The model under review builds one solid part; all positions refer to its coordinate system, in mm. Give positions to 0.01 mm unless a question says otherwise; leave off trailing zeros. Loops run counter-clockwise (first coordinate to the right, second up) from the corner with the lowest first, then second, coordinate; pieces in that order, holes last. Notation, with made-up numbers: M 81.5,56 L 136.5,56 A19 ccw 136.5,83 Z; hole C 20.25,71 d1. An arc over 180 degrees is marked long. Write item = value, one per line. Start each with the question number.
1. Wall thickness on line 1 along Y through (x, z) = (-12.5, 0.6); line 2 along X through (y, z) = (6, 1.4); line 3 along Y through (x, z) = (12, 0.5): over which ranges is each line inside the solid? List them lowest first. Write a range as from..to.
2. We need section D-D on y = 4. Give the boundary of the cut face in (x, z).
3. For pin 1 (8 mm diameter, centred on x = 12.5, y = 0, fed in from -Z); pin 2 (1.1 mm diameter, centred on x = -4.5, z = 0.5, fed in from +Y); pin 3 (1.5 mm diameter, centred on y = -2, z = 3, fed in from +X); pin 4 (1.5 mm diameter, centred on x = -14.5, z = -0.5, fed in from +Y), all flat-tipped, find the tip position at first contact; note any pin that passes through.
4. We need section A-A on y = 0. Give the boundary of the cut face in (x, z).
5. We need section C-C on z = -0.35. Give the boundary of the cut face in (x, y).
6. We need section B-B on x = 12.5. Count the separate pieces of the cut face and the enclosed holes in it, then the cut area to 3 significant figures.
7. Draft analysis for pull direction Z (two halves, no side actions). For faces 1 (the face through (0, 0, 0)), 2 (the face through (14.07, 6.536, 1.827)), 3 (the face through (9, 9, 0)), state which applies: pulls with the +Z half, pulls with the -Z half, needs draft (parallel to the pull), parting line crosses it, or undercut.
from build123d import *

# Parameters (mm, degrees)
SKETCH_1_W      = 38
SKETCH_1_H      = 12
SKETCH_1_R      = 2.5
EXTRUDE_1_DEPTH = 1
SKETCH_3_R      = 2.50184692
SKETCH_3_R_2    = 1.5
EXTRUDE_4_DEPTH = 10
EXTRUDE_START   = 10
SKETCH_4_R      = 2.50184692
SKETCH_4_R_2    = 1.50184692
EXTRUDE_5_DEPTH = 10


with BuildPart() as part:
    # 草图1 → 凸台-拉伸1 (new body)
    with BuildSketch(Plane.XY):
        Rectangle(SKETCH_1_W, SKETCH_1_H)
        with Locations((12.5, 0)):
            Circle(SKETCH_1_R, mode=Mode.SUBTRACT)
        with Locations((-12.5, 0)):
            Circle(SKETCH_1_R, mode=Mode.SUBTRACT)
    extrude(amount=EXTRUDE_1_DEPTH)

    # 草图3 → 凸台-拉伸4 (add)
    with BuildSketch(Plane.ZY.offset(9)):
        with Locations((1.50184692, 8.00184692)):
            Circle(SKETCH_3_R)
        with Locations((1.50184692, 8.00184692)):
            Circle(SKETCH_3_R_2, mode=Mode.SUBTRACT)
    extrude(amount=EXTRUDE_4_DEPTH)

    # 草图4 → 凸台-拉伸5 (add)
    with BuildSketch(Plane(origin=(9, 0, 0), x_dir=(0, 0, -1), z_dir=(1, 0, 0)).offset(EXTRUDE_START)):
        with Locations((-1.50184692, 8.00184692)):
            Circle(SKETCH_4_R)
        with Locations((-1.50184692, 8.00184692)):
            Circle(SKETCH_4_R_2, mode=Mode.SUBTRACT)
    extrude(amount=-EXTRUDE_5_DEPTH)


solid = part.part
Final values:
q1.line_1 = -6..-2.5, 2.5..6.8, 9.2..10.34
q1.line_2 = -19..-9, 9..19
q1.line_3 = -6..-2.45, 2.45..6.88, 9.12..10.29
q2.outline = M -19,0 L 19,0 L 19,1 L -19,1 Z
q3.pin_1 = 0
q3.pin_2 = 6
q3.pin_3 = through
q3.pin_4 = 10.17
q4.outline = M -19,0 L -15,0 L -15,1 L -19,1 Z; M -10,0 L 10,0 L 10,1 L -10,1 Z; M 15,0 L 19,0 L 19,1 L 15,1 Z
q5.outline = M -19,6.32 L -9,6.32 L -9,9.68 L -19,9.68 Z; M 9,6.32 L 19,6.32 L 19,9.68 L 9,9.68 Z
q6.separate_pieces = 2
q6.enclosed_holes = 1
q6.area = 19.3 mm²
q7.face_1 = pulls with the -Z half
q7.face_2 = undercut
q7.face_3 = needs draft
